The listing builds one solid part. Answer for the finished solid, in the listing's coordinates (mm). A direction names the side the tool comes from. Give positions to 0.01 mm unless a question says otherwise; leave off trailing zeros. Write each loop counter-clockwise with the first axis right and the second up, starting at its lowest first coordinate (ties: lowest second). Pieces come first, ordered by that corner, then holes. Notation, with made-up numbers: (-1.5, -34) -> (9.5, -34) arc R5 ccw to (9.5, -27) -> close; hole circle Ø9 at (69.5, -5). An arc over 180 degrees is marked (long way). Put each result on its own line as item: value. Start each with the question number.
1) A cutting plane is placed at A-A (z = -2.5). Write down the section's boundary in (x, y) (3 decimals), then the cut area to 3 significant figures.
2) Find the intervals of material crossed by line 1 along X through (y, z) = (1.45, -27) (3 decimals); line 2 along X through (y, z) = (1.9, -13.5) (3 decimals); line 3 along Z through (x, y) = (12.5, 2.35), in increasing order. Write a range as from..to.
3) A cutting plane is placed at D-D (y = 2). Give the number of separate pieces and of enclosed holes in the cut face, then the cut area to 3 significant figures.
4) For a pull along Z with two mould halves and no side action, classify faces 1 (the flat face through (-11.262, 2, -20)), 2 (the flat face through (4, 2, -39)), 3 (the flat face through (-19.375, 2, -19)) as released by +Z, released by -Z, zero draft, split by the parting line, or undercut.
5) Flat-ended cylindrical pins translate along their axes: pin 1 Ø0.9 at (x, y) = (-0.5, 1.5) entering from -Z; pin 2 Ø0.5 at (x, y) = (10.5, 1) entering from -Z. Find the tip coordinate at first contact, or state that the pin passes through.
6) For faces 4 (the flat face through (0, 0, -20)), 5 (the flat face through (1.65, 2, -27)), 6 (the flat face through (-1.65, 2, -34)), determine the directions among +Z, -Z, +X, -X, +Y, -Y from which every point of the face is accessible in a straight line to the end or side of a thin tool.
7) A cutting plane is placed at C-C (z = -36). Write down the section's boundary in (x, y) (3 decimals).
8) A cutting plane is placed at B-B (x = -0.5). Write down the section's boundary in (y, z).
from build123d import *

# Parameters (mm, degrees)
BOSS_EXTRUDE1_DEPTH                = 3.05
FILLET3_R                          = 0.5
SKETCH2_W                          = 3.3
SKETCH2_H                          = 47
SKETCH2_H_2                        = 1
CUT_EXTRUDE1_DEPTH                 = 44.654245212
SKETCH6_W                          = 2
SKETCH6_H                          = 21.5
CUT_EXTRUDE2_DEPTH                 = 44.654245212
FILLET4_R                          = 0.5
M3_CLEARANCE_HEAD_MOUNTING_HOLES_D = 3.4


with BuildPart() as part:
    # Sketch1 → Boss-Extrude1 (new body)
    with BuildSketch(Plane(origin=(0, 0, 0), x_dir=(1, 0, 0), z_dir=(0, 1, 0))):
        Polygon((-19.375, 0), (-19.375, 39), (-12.375, 39), (-15.261751346, 34), (-5.261751346, 34), (-8.148502692, 39), (8.148502692, 39), (5.261751346, 34), (15.261751346, 34), (12.375, 39), (19.375, 39), (19.375, 0), align=None)
    extrude(amount=BOSS_EXTRUDE1_DEPTH)

    # Fillet3
    fillet3_edges = [part.edges().sort_by_distance(p)[0] for p in [
        (-12.375, 1.525, -39),
        (-15.261751346, 1.525, -34),
        (-5.261751346, 1.525, -34),
        (-8.148502692, 1.525, -39),
        (8.148502692, 1.525, -39),
        (5.261751346, 1.525, -34),
        (15.261751346, 1.525, -34),
        (12.375, 1.525, -39),
    ]]
    fillet(fillet3_edges, radius=FILLET3_R)

    # Sketch2 → Cut-Extrude1 (cut, through all)
    with BuildSketch(Plane(origin=(0, 3.05, 0), x_dir=(1, 0, 0), z_dir=(0, 1, 0))):
        with Locations((0, 52.5)):
            Rectangle(SKETCH2_W, SKETCH2_H)
        with Locations((0, 27.3)):
            Rectangle(SKETCH2_W, SKETCH2_H_2)
    extrude(amount=-CUT_EXTRUDE1_DEPTH, mode=Mode.SUBTRACT)

    # Sketch6 → Cut-Extrude2 (cut, through all)
    with BuildSketch(Plane(origin=(0, 3.05, 0), x_dir=(1, 0, 0), z_dir=(0, 1, 0))):
        with Locations((-10.261751346, 20.25)):
            Rectangle(SKETCH6_W, SKETCH6_H)
        with Locations((10.261751346, 20.25)):
            Rectangle(SKETCH6_W, SKETCH6_H)
    extrude(amount=-CUT_EXTRUDE2_DEPTH, mode=Mode.SUBTRACT)

    # Fillet4
    fillet4_edges = [part.edges().sort_by_distance(p)[0] for p in [
        (-11.261751346, 1.525, -9.5),
        (-11.261751346, 1.525, -31),
        (-9.261751346, 1.525, -31),
        (-9.261751346, 1.525, -9.5),
        (11.261751346, 1.525, -31),
        (11.261751346, 1.525, -9.5),
        (9.261751346, 1.525, -9.5),
        (9.261751346, 1.525, -31),
    ]]
    fillet(fillet4_edges, radius=FILLET4_R)

    # M3 Clearance Head Mounting Holes (through all)
    with Locations(Plane(origin=(0, 3.05, 0), x_dir=(1, 0, 0), z_dir=(0, 1, 0))):
        with Locations((-12.5, 2.5), (12.5, 2.5)):
            Hole(M3_CLEARANCE_HEAD_MOUNTING_HOLES_D / 2)


solid = part.part
Reply:
1. outline: (-19.375, 0) -> (-14.2, 0) -> (-14.2, 3.05) -> (-19.375, 3.05) -> close; (-10.8, 0) -> (10.8, 0) -> (10.8, 3.05) -> (-10.8, 3.05) -> close; (14.2, 0) -> (19.375, 0) -> (19.375, 3.05) -> (14.2, 3.05) -> close
1. area: 97.4 mm2
2. line 1: x = -19.375..-11.262, -9.262..-1.65, 1.65..9.262, 11.262..19.375
2. line 2: x = -19.375..-11.262, -9.262..9.262, 11.262..19.375
2. line 3: z = -34..-4.2, -0.8..0
3. separate pieces: 1
3. enclosed holes: 5
3. area: 1,300 mm2
4. face 1: undercut
4. face 2: released by -Z
4. face 3: zero draft
5. pin 1: stops at z = -29
5. pin 2: stops at z = -34
6. face 4: +Z, -Z, +X, -X, -Y
6. face 5: +Y, -Y
6. face 6: -Z, +Y, -Y
7. outline: (-19.375, 0) -> (-14.107, 0) -> (-14.107, 3.05) -> (-19.375, 3.05) -> close; (-6.416, 0) -> (-1.65, 0) -> (-1.65, 3.05) -> (-6.416, 3.05) -> close; (1.65, 0) -> (6.416, 0) -> (6.416, 3.05) -> (1.65, 3.05) -> close; (14.107, 0) -> (19.375, 0) -> (19.375, 3.05) -> (14.107, 3.05) -> close
8. outline: (0, -29) -> (3.05, -29) -> (3.05, -27.8) -> (0, -27.8) -> close; (0, -26.8) -> (3.05, -26.8) -> (3.05, 0) -> (0, 0) -> close
